Part model, mm, in its own coordinate system. Face numbers are marked on the shaded views. Give positions to 0.01 mm unless a question says otherwise; leave off trailing zeros. Write each loop counter-clockwise with the first axis right and the second up, starting at its lowest first coordinate (ties: lowest second). Pieces come first, ordered by that corner, then holes. Notation, with made-up numbers: (23, 66.5) - (32, 66.5) arc R18 cw to (32, 78.5) - close; hole circle Ø7 at (-37, 53.25). An arc over 180 degrees is marked (long way). Answer as a JSON object with one key per item and string values. Group by question number.
```python
from build123d import *

# Parameters (mm, degrees)
SKETCH1_R           = 47
BOSS_EXTRUDE2_DEPTH = 8.5
SKETCH2_R           = 32.55
CUT_EXTRUDE1_DEPTH  = 7
SKETCH3_R           = 31
BRAIN_DEPTH         = 67.835619246
SKETCH4_R           = 1.7
SCREW_HOLES_DEPTH   = 68.009327709


with BuildPart() as part:
    # Sketch1 → Boss-Extrude2 (new body)
    with BuildSketch(Plane.XY):
        Circle(SKETCH1_R)
    extrude(amount=BOSS_EXTRUDE2_DEPTH)

    # Sketch2 → Cut-Extrude1 (cut)
    with BuildSketch(Plane.XY.offset(8.5)):
        Circle(SKETCH2_R)
    extrude(amount=-CUT_EXTRUDE1_DEPTH, mode=Mode.SUBTRACT)

    # Sketch3 → Brain (cut, through all)
    with BuildSketch(Plane.XY.offset(1.5)):
        Circle(SKETCH3_R)
    extrude(amount=-BRAIN_DEPTH, mode=Mode.SUBTRACT)

    # Sketch4 → Screw Holes (cut, through all)
    with BuildSketch(Plane.XY):
        with Locations((-43.25, 0)):
            Circle(SKETCH4_R)
        with Locations((-21.625, 37.455598714)):
            Circle(SKETCH4_R)
        with Locations((21.625, 37.455598714)):
            Circle(SKETCH4_R)
        with Locations((43.25, 0)):
            Circle(SKETCH4_R)
        with Locations((21.625, -37.455598714)):
            Circle(SKETCH4_R)
        with Locations((-21.625, -37.455598714)):
            Circle(SKETCH4_R)
    extrude(amount=SCREW_HOLES_DEPTH, mode=Mode.SUBTRACT)


solid = part.part
```
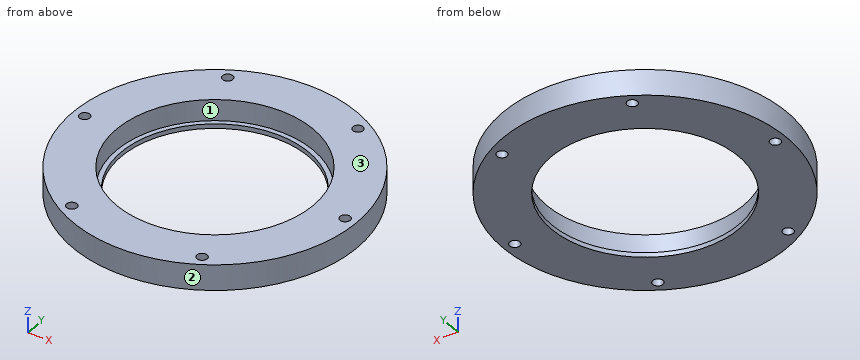
1) Saw through at C-C (y = -10.5). List the corners of the cut face in (x, z), and give its area (3 significant figures).
2) Saw through at B-B (x = 0). List the corners of the cut face in (y, z), and give its area (3 significant figures).
3) Drop flat-ended pins along their axis: P1, Ø1, axis at x = -24, y = 15.5, coming from the +Z side; P2, Ø1, axis at y = -22, z = 5, coming from the +X side; P3, Ø4, axis at y = 8.5, z = 7, coming from the +X side; P4, Ø4, axis at y = -4, z = 2, coming from the -X side. Give the stop position or say it passes through.
4) Drill centre lines: line 1 along Y through (x, z) = (21.5, 3); line 2 along X through (y, z) = (-1, 4.25); line 3 along Y through (x, z) = (11, 2). Where is each one in solid material? Low to high. Write a range as from..to.
5) Saw through at A-A (y = 0). List the corners of the cut face in (x, z), and give its area (4 significant figures).
6) Two-plate mould, pull along X, no slides. Class the marked faces 1, 2 and 3: +X half, -X half, draft (parallel to the pull), parting line (faces both ways), or undercut.
7) Saw through at D-D (z = 6). List the corners of the cut face in (x, y) (3 decimals), and give its area (3 significant figures).
Checks:
{
 "1": {"outline": "(-45.81, 0) - (-29.17, 0) - (-29.17, 1.5) - (-30.81, 1.5) - (-30.81, 8.5) - (-45.81, 8.5) - close; (29.17, 0) - (45.81, 0) - (45.81, 8.5) - (30.81, 8.5) - (30.81, 1.5) - (29.17, 1.5) - close", "area": "260 mm2"},
 "2": {"outline": "(-47, 0) - (-31, 0) - (-31, 1.5) - (-32.55, 1.5) - (-32.55, 8.5) - (-47, 8.5) - close; (31, 0) - (47, 0) - (47, 8.5) - (32.55, 8.5) - (32.55, 1.5) - (31, 1.5) - close", "area": "250 mm2"},
 "3": {"P1": "through", "P2": "x = 41.79", "P3": "x = 46.55", "P4": "x = -46.96"},
 "4": {"line 1": "-41.79..-39.15, -35.76..-24.44, 24.44..35.76, 39.15..41.79", "line 2": "-46.99..-44.62, -41.88..-32.53, 32.53..41.88, 44.62..46.99", "line 3": "-45.69..-30.63, 30.63..45.69"},
 "5": {"outline": "(-47, 0) - (-44.95, 0) - (-44.95, 8.5) - (-47, 8.5) - close; (-41.55, 0) - (-31, 0) - (-31, 1.5) - (-32.55, 1.5) - (-32.55, 8.5) - (-41.55, 8.5) - close; (31, 0) - (41.55, 0) - (41.55, 8.5) - (32.55, 8.5) - (32.55, 1.5) - (31, 1.5) - close; (44.95, 0) - (47, 0) - (47, 8.5) - (44.95, 8.5) - close", "area": "192.5 mm2"},
 "6": {"face 1": "undercut", "face 2": "parting line", "face 3": "draft"},
 "7": {"outline": "circle Ø94 at (0, 0); hole circle Ø3.4 at (-43.25, 0); hole circle Ø65.1 at (0, 0); hole circle Ø3.4 at (-21.625, -37.456); hole circle Ø3.4 at (-21.625, 37.456); hole circle Ø3.4 at (21.625, -37.456); hole circle Ø3.4 at (21.625, 37.456); hole circle Ø3.4 at (43.25, 0)", "area": "3,560 mm2"}
}
